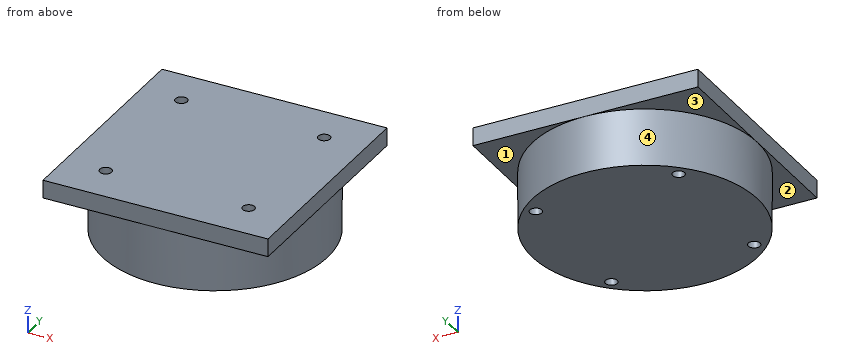
```python
from build123d import *

# Parameters (mm, degrees)
SKETCH1_R           = 25
BOSS_EXTRUDE1_DEPTH = 12.7
SKETCH2_W           = 50
SKETCH2_H           = 50
BOSS_EXTRUDE2_DEPTH = 4
SKETCH3_R           = 1.32
CUT_EXTRUDE1_DEPTH  = 17.7


with BuildPart() as part:
    # Sketch1 → Boss-Extrude1 (new body)
    with BuildSketch(Plane.XY):
        Circle(SKETCH1_R)
    extrude(amount=BOSS_EXTRUDE1_DEPTH)

    # Sketch2 → Boss-Extrude2 (add)
    with BuildSketch(Plane.XY.offset(12.7)):
        Rectangle(SKETCH2_W, SKETCH2_H)
    extrude(amount=BOSS_EXTRUDE2_DEPTH)

    # Sketch3 → Cut-Extrude1 (cut, through all)
    with BuildSketch(Plane.XY.offset(16.7)):
        with Locations((-15.875, 15.875)):
            Circle(SKETCH3_R)
        with Locations((15.875, 15.875)):
            Circle(SKETCH3_R)
        with Locations((15.875, -15.875)):
            Circle(SKETCH3_R)
        with Locations((-15.875, -15.875)):
            Circle(SKETCH3_R)
    extrude(amount=-CUT_EXTRUDE1_DEPTH, mode=Mode.SUBTRACT)


solid = part.part
```
CAD build for the part. Positions are in the model's coordinates, mm. Face numbers are marked on the shaded views. A direction names the side the tool comes from. Round coordinates to 2 decimals unless told otherwise and drop trailing zeros. Loops run counter-clockwise (first coordinate to the right, second up) from the corner with the lowest first, then second, coordinate; pieces in that order, holes last. Notation, with made-up numbers: (6.5, 30.5) - (25.5, 30.5) arc R15 ccw to (25.5, 46.5) - close; hole circle Ø1 at (-13, 26.25). An arc over 180 degrees is marked (long way). Return JSON: item names as keys, results as strings. Group by question number.
Q1. Flat gauge pins, fed straight in: pin 1 Ø2 at (y, z) = (-5.5, 9.5) entering from -X; pin 2 Ø1 at (x, y) = (-18, 20) entering from -Z; pin 3 Ø2.5 at (x, y) = (-15.875, 15.875) entering from -Z; pin 4 Ø8 at (y, z) = (-8, 6.5) entering from +X. Where does each tip first touch, or does it go through?
Q2. Tool access for the marked faces 1, 2, 3 and 4: list every direction of +Z, -Z, +X, -X, +Y, -Y with a clear straight run to the whole face (end or side of a thin tool).
Q3. Drill centre lines: line 1 along Y through (x, z) = (17, 10.75); line 2 along Y through (x, z) = (-16, 6.25). Where is each one in solid material? Low to high. Write a range as [from, to].
Q4. Band-saw the part on B-B on y = 10.5. Give the cut face in (x, z).
Q5. Band-saw the part on C-C on z = 11.25. Give the cut face in (x, y) (3 decimals), plus the area to 3 significant figures.
Q6. Band-saw the part on A-A on x = -12.5. Give the cut face in (y, z).
Solutions:
{
 "1": {"pin 1": "stops at x = -24.59", "pin 2": "stops at z = 12.7", "pin 3": "passes through", "pin 4": "stops at x = 24.68"},
 "2": {"face 1": "-Z, +X, +Y", "face 2": "-Z, -X, -Y", "face 3": "-Z, -X, +Y", "face 4": "-Z"},
 "3": {"line 1": "y = [-18.33, -16.57], [-15.18, 15.18], [16.57, 18.33]", "line 2": "y = [-19.21, -17.19], [-14.56, 14.56], [17.19, 19.21]"},
 "4": {"outline": "(-25, 12.7) - (-22.69, 12.7) - (-22.69, 0) - (22.69, 0) - (22.69, 12.7) - (25, 12.7) - (25, 16.7) - (-25, 16.7) - close"},
 "5": {"outline": "circle Ø50 at (0, 0); hole circle Ø2.64 at (-15.875, -15.875); hole circle Ø2.64 at (-15.875, 15.875); hole circle Ø2.64 at (15.875, -15.875); hole circle Ø2.64 at (15.875, 15.875)", "area": "1,940 mm^2"},
 "6": {"outline": "(-25, 12.7) - (-21.65, 12.7) - (-21.65, 0) - (21.65, 0) - (21.65, 12.7) - (25, 12.7) - (25, 16.7) - (-25, 16.7) - close"}
}
